Read the model definition and answer for the solid it produces. Units are mm, in the model's axes. A direction names the side the tool comes from. Coordinates: 2 decimals unless noted, no trailing zeros. Loops run counter-clockwise (first coordinate to the right, second up) from the corner with the lowest first, then second, coordinate; pieces in that order, holes last. Notation, with made-up numbers: (-22, 50.25) -> (-1, 50.25) arc R16 cw to (-1, 55.25) -> close; hole circle Ø3 at (72, 19). An arc over 180 degrees is marked (long way). Answer as a JSON object with one key per item and string values. Group by question number.
Q1. For faces 4 (the flat face through (-22.5, -81, -20)), 5 (the flat face through (22.5, -81, -20)), 6 (the flat face through (0, -87, -10)), determine the directions among +Z, -Z, +X, -X, +Y, -Y from which every point of the face is accessible in a straight line to the end or side of a thin tool.
Q2. The part is cut by section B-B on y = -130. Write down the section's boundary in (x, z).
Q3. The part is cut by section A-A on x = 0. Write down the section's boundary in (y, z).
Q4. Each of these flat-tipped pins is pushed along its axis until it touches: P1, Ø9, axis at x = 30.5, z = -17.5, coming from the -Y side; P2, Ø10, axis at y = -102, z = -23.5, coming from the -X side; P3, Ø16, axis at y = -65, z = -16.5, coming from the +X side. Where does it stop, or does it pass through?
Q5. The part is cut by section C-C on z = -27.25. Write down the section's boundary in (x, y).
Q6. The part is cut by section D-D on x = 45.5. Write down the section's boundary in (y, z).
Q7. Straight lines are drawn through the part: line 1 along Y through (x, z) = (0, -25.75); line 2 along Y through (x, z) = (0.5, -22); line 3 along X through (y, z) = (-130, -25.25). For each, find the intervals that lie inside material, in ascending order. Write a range as [from, to].
Q8. Determine the mould class of faces 1 (the cylindrical face through (-2, -10, -15)), 2 (the flat face through (2, -12, 0)), 3 (the flat face through (-2, 0, -15)) for opening direction Z: released by +Z, released by -Z, zero draft, split by the parting line, or undercut.
from build123d import *

# Parameters (mm, degrees)
F1_DEPTH      = 25
F3_DEPTH      = 22.5
F3_DEPTH_BACK = 22.5
F4_R          = 15
F6_D          = 5
F8_D          = 5


with BuildPart() as f1:
    # F0 (on Front) → F1 (new body)
    with BuildSketch(Plane.XZ):
        Polygon((-22.5, -20), (0, -20), (0, 0), (-122.5, 0), (-122.5, -30), (-22.5, -30), align=None)
        Polygon((0, 0), (0, -20), (22.5, -20), (22.5, -30), (122.5, -30), (122.5, 0), align=None)
    extrude(amount=F1_DEPTH)

    # F2 (on Right) → F3 (join, two sides)
    with BuildSketch(Plane.YZ) as f3_sk:
        Polygon((-25, -10), (-150, -10), (-150, -30), (0, -30), (0, -20), (-25, -20), align=None)
    extrude(amount=F3_DEPTH)
    extrude(f3_sk.sketch, amount=-F3_DEPTH_BACK)

    # F4
    f4_edges = [f1.edges().sort_by_distance(p)[0] for p in [
        (-22.5, -150, -20),
        (22.5, -150, -20),
    ]]
    fillet(f4_edges, radius=F4_R)

    # F6 (through all)
    with Locations(Plane.XY):
        with Locations((0, -130)):
            Hole(F6_D / 2)

    # F8 (through all)
    with Locations(Plane.YZ.offset(122.5)):
        with Locations((-12.5, -15)):
            Hole(F8_D / 2)


solid = f1.part
Final values:
{
 "1": {"face 4": "+Z, -Z, -X, -Y", "face 5": "+Z, -Z, +X, -Y", "face 6": "+Z, +X, -X, -Y"},
 "2": {"outline": "(-22.5, -30) -> (-2.5, -30) -> (-2.5, -10) -> (-22.5, -10) -> close; (2.5, -30) -> (22.5, -30) -> (22.5, -10) -> (2.5, -10) -> close"},
 "3": {"outline": "(-150, -30) -> (-132.5, -30) -> (-132.5, -10) -> (-150, -10) -> close; (-127.5, -30) -> (0, -30) -> (0, 0) -> (-25, 0) -> (-25, -10) -> (-127.5, -10) -> close; hole circle Ø5 at (-12.5, -15)"},
 "4": {"P1": "stops at y = -25", "P2": "stops at x = -22.5", "P3": "stops at x = 22.5"},
 "5": {"outline": "(-122.5, -25) -> (-22.5, -25) -> (-22.5, -135) arc R15 ccw to (-7.5, -150) -> (7.5, -150) arc R15 ccw to (22.5, -135) -> (22.5, -25) -> (122.5, -25) -> (122.5, 0) -> (-122.5, 0) -> close; hole circle Ø5 at (0, -130)"},
 "6": {"outline": "(-25, -30) -> (0, -30) -> (0, 0) -> (-25, 0) -> close; hole circle Ø5 at (-12.5, -15)"},
 "7": {"line 1": "y = [-150, -132.5], [-127.5, 0]", "line 2": "y = [-150, -132.45], [-127.55, 0]", "line 3": "x = [-22.5, -2.5], [2.5, 22.5]"},
 "8": {"face 1": "undercut", "face 2": "released by +Z", "face 3": "zero draft"}
}
